from build123d import *

# Parameters (mm, degrees)
F0_W     = 5.95
F0_H     = 2.95
F1_DEPTH = 3.175
F2_R     = 6.35


with BuildPart() as f1:
    # F0 (on Front) → F1 (new body)
    with BuildSketch(Plane.XZ):
        with BuildLine():
            Line((0, 28.642999), (-6.35, 0))
            ThreePointArc((-6.35, 0), (0, -6.217982), (6.35, 0))
            Line((6.35, 0), (7.62, 28.642999))
            Line((7.62, 28.642999), (-2.570709, 44.594768))
            Line((-2.570709, 44.594768), (2.537907, 52.743887))
            Line((2.537907, 52.743887), (0, 65.412782))
            Line((0, 65.412782), (-2.54, 52.88969))
            Line((-2.54, 52.88969), (-8.920709, 44.594768))
            Line((-8.920709, 44.594768), (0, 28.642999))
        make_face()
        with Locations((-0.025, 0.025)):
            Rectangle(F0_W, F0_H, mode=Mode.SUBTRACT)
    extrude(amount=F1_DEPTH)

    # F2
    f2_edges = [f1.edges().sort_by_distance(p)[0] for p in [
        (2.537907, -1.5875, 52.743887),
        (-2.570709, -1.5875, 44.594768),
        (7.62, -1.5875, 28.642999),
        (0, -1.5875, 28.642999),
        (-8.920709, -1.5875, 44.594768),
        (-2.54, -1.5875, 52.88969),
    ]]
    fillet(f2_edges, radius=F2_R)


solid = f1.part
Design review of the part built by this model. Coordinates are the model's own, in mm. A direction names the side the tool comes from. Give positions to 0.01 mm unless a question says otherwise; leave off trailing zeros. Loops run counter-clockwise (first coordinate to the right, second up) from the corner with the lowest first, then second, coordinate; pieces in that order, holes last. Notation, with made-up numbers: M 89,15 L 140,15 A30 ccw 140,53 Z; hole C 75.25,25.5 d6. An arc over 180 degrees is marked long. Answer as a JSON object with one key per item and string values.
Item 1: Wall thickness on line 1 along X through (y, z) = (-2.95, 1); line 2 along X through (y, z) = (-2.9, 17.5); line 3 along X through (y, z) = (-1.75, 48): over which ranges is each line inside the solid? List them lowest first.
Output values:
{"line 1": "x = -6.13 to -3, 2.95 to 6.39", "line 2": "x = -2.47 to 7.13", "line 3": "x = -6.3 to -0.44"}
Item 2: For P1, Ø1, axis at y = -1, z = 22, coming from the -X side; P2, Ø1.5, axis at x = -3, y = -1, coming from the -Z side, all flat-tipped, find the tip position at first contact; note any pin that passes through.
Output values:
{"P1": "stops at x = -1.58", "P2": "stops at z = -5.81"}
Item 3: Mouldability with a two-part tool opening along X and no side actions: class faces 1 (the face through (0, -2, 1.5)), 2 (the face through (-3.4, -1.6, 13.3)), 3 (the face through (1.035, -1.565, 60.246)), 4 (the face through (-3, -2, 0)) as pulls with the +X half, pulls with the -X half, needs draft (parallel to the pull), parting line crosses it, or undercut.
Output values:
{"face 1": "undercut", "face 2": "pulls with the -X half", "face 3": "pulls with the +X half", "face 4": "undercut"}
Item 4: We need section B-B (z = 7). State the section outline as (x, y) points (3 decimals), and give its area (3 significant figures).
Output values:
{"outline": "M -4.798,-3.175 L 6.66,-3.175 L 6.66,0 L -4.798,0 Z", "area": "36.4 mm2"}
Item 5: We need section C-C (z = 38). State the section outline as (x, y) points (3 decimals).
Output values:
{"outline": "M -5.233,-3.175 L 1.642,-3.175 L 1.642,0 L -5.233,0 Z"}
Item 6: We need section A-A (y = -1.6). State the section outline as (x, z) points, and give its area (3 significant figures).
Output values:
{"outline": "M -6.88,40.94 L -1.18,30.75 A6.35 cw -0.52,26.28 L -6.35,0 A6.35 ccw 6.35,0 L 7.53,26.64 A6.35 ccw 6.54,30.34 L -0.41,41.21 A6.35 cw -0.44,48 L 1.2,50.6 A6.35 ccw 2.04,55.22 L 0,65.41 L -2.25,54.33 A6.35 cw -3.44,51.72 L -6.37,47.91 A6.35 ccw Z; hole M -3,-1.45 L 2.95,-1.45 L 2.95,1.5 L -3,1.5 Z", "area": "525 mm2"}
Item 7: Machinability: for faces 5 (the face through (2.95, -2, 0)), 6 (the face through (-4.07, -1.57, 35.92)), 7 (the face through (0.368, -1.565, 49.283)), which of the approach directions +Z, -Z, +X, -X, +Y, -Y give a long, thin tool a straight path to every point of the face, cutting with its end or side? Answer none if there is none.
Output values:
{"face 5": "+Y, -Y", "face 6": "-X, +Y, -Y", "face 7": "+X, +Y, -Y"}
